Geometry: final body of the model. Coordinates: model frame, mm. A direction names the side the tool comes from. Round coordinates to 2 decimals unless told otherwise and drop trailing zeros. Write each loop counter-clockwise with the first axis right and the second up, starting at its lowest first coordinate (ties: lowest second). Pieces come first, ordered by that corner, then holes. Notation, with made-up numbers: M 85.25,3 L 126.25,3 A22 ccw 126.25,22 Z; hole C -33,-17.75 d4. An arc over 180 degrees is marked long. Use one line per item in the form item = value. Start each with the question number.
Item 1: Section query C-C (x = 5). Return loops of the section in (y, z).
Item 2: Pull-direction query (X, two-part tool) for faces 1 (the cylindrical face through (-1.38, 6.2, 64.86)), 2 (the cylindrical face through (-0.748, -2.374, 118.694)), 3 (the flat face through (3, 0, 0)); classes: pulls with the +X half, pulls with the -X half, needs draft (parallel to the pull), parting line crosses it, or undercut.
Item 3: Pin query (flat end, axial travel): pin 1 Ø1 at (x, z) = (-3.5, 43.5) entering from -Y; pin 2 Ø2 at (y, z) = (2.5, 49) entering from +X; pin 3 Ø1 at (x, z) = (3.5, 71.5) entering from +Y. Return the tip coordinate at first contact, or that it passes through.
Item 4: Ray query, probe 1 along Y at (x, z) = (0, 119); probe 2 along X at (y, z) = (1, 122); probe 3 along X at (y, z) = (-4.5, 113). Return the intervals inside material, ascending.
Item 5: Section query B-B (z = 61.5). Return loops of the section in (x, y).
Item 6: Reachability of faces 4 (the flat face through (3, 0, 131.572)), 5 (the cylindrical face through (-0.748, 2.374, 12.878)) from +Z, -Z, +X, -X, +Y, -Y: full face, straight path, thin tool, end or side. Return the list, or none.
Item 7: Section query A-A (z = 14). Return loops of the section in (x, y).
Autodesk Inventor part; units mm, degrees
ref_plane "YZ Plane" through (0, 0, 0) normal (1, 0, 0) x (0, 1, 0)
ref_plane "XZ Plane" through (0, 0, 0) normal (0, 1, 0) x (-1, 0, 0)
ref_plane "XY Plane" through (0, 0, 0) normal (0, 0, 1) x (1, 0, 0)
sketch "Sketch1" plane through (0, 0, 0) normal (0, 0, 1) x (1, 0, 0)
  circle A0 centre (0, 0) radius 6.35
  dimension "d0" = 12.7
extrude "Extrusion1" add sketch "Sketch1" along normal blind 131.572
sketch "Sketch2" plane through (0, 0, 131.572) normal (0, 0, 1) x (1, 0, 0)
  circle A0 centre (0, 0) radius 6.35
hole "Hole1" at (0, 0, 131.572) direction (0, 0, -1) diameter 4.9784 depth 25.4 tip angle 118
sketch "Sketch3" plane through (0, 0, 0) normal (0, 0, -1) x (-1, 0, 0)
  circle A0 centre (0, 0) radius 6.35
hole "Hole2" at (0, 0, 0) direction (0, 0, 1) diameter 4.9784 depth 25.4 tip angle 118
properties part number "Axle Nick" material "Stainless Steel"
Working result:
q1.outline = M -3.91,0 L 3.91,0 L 3.91,131.57 L -3.91,131.57 Z
q2.face_1 = parting line crosses it
q2.face_2 = undercut
q2.face_3 = needs draft
q3.pin_1 = -5.6
q3.pin_2 = 6.17
q3.pin_3 = 5.6
q4.probe_1 = -6.35 to -2.49, 2.49 to 6.35
q4.probe_2 = -6.27 to -2.28, 2.28 to 6.27
q4.probe_3 = -4.48 to 4.48
q5.outline = C 0,0 d12.7
q6.face_4 = +Z, +X, -X, +Y, -Y
q6.face_5 = -Z
q7.outline = C 0,0 d12.7; hole C 0,0 d4.98
